Input: part model. Units: mm. Frame: model coordinates. Face numbers are marked on the shaded views. Round coordinates to 2 decimals unless told otherwise and drop trailing zeros. Loops run counter-clockwise (first coordinate to the right, second up) from the corner with the lowest first, then second, coordinate; pieces in that order, holes last. Notation, with made-up numbers: M 78,52 L 85,52 A36 cw 85,88 Z; hole C 77.5,13.5 d4. An arc over 180 degrees is marked long. Use one line per item in the form item = value. Start each with the question number.
Q1. First-contact query: P1, Ø2, axis at x = -1, y = -0.5, coming from the +Z side; P2, Ø1, axis at x = -2, y = 1.5, coming from the -Z side. Flat tips, straight axial feed; report the tip coordinate or a pass-through.
Q2. Section query A-A, the plane z = 0. Output: boundary loops of the cut face in (x, y) (3 decimals).
Q3. Section query B-B, the plane x = 0. Output: boundary loops of the cut face in (y, z) (3 decimals).
Q4. Section query C-C, the plane y = -1.5. Output: boundary loops of the cut face in (x, z).
Q5. Section query D-D, the plane y = 0.25. Output: boundary loops of the cut face in (x, z), and give its area (3 significant figures).
Q6. Ray query, line 1 along Z through (x, y) = (4.5, 2.5); line 2 along X through (y, z) = (-1.25, 2.5); line 3 along Z through (x, y) = (3.75, -1.5). Return the intervals inside material, ascending.
Q7. Mould query, pull axis Z, two halves, no side actions, for the marked faces 1 and 2. Classes: pulls with the +Z half, pulls with the -Z half, needs draft (parallel to the pull), parting line crosses it, or undercut.
```python
from build123d import *

# Parameters (mm, degrees)
SZKIC1_R                    = 8
DODANIE_WYCI_GNI_CIE1_DEPTH = 3.375
ZAOKR_GLENIE1_R             = 0.2


with BuildPart() as part:
    # Szkic1 → Dodanie-wyciągnięcie1 (new body, symmetric)
    with BuildSketch(Plane(origin=(0, 0, 0), x_dir=(1, 0, 0), z_dir=(0, 1, 0))):
        Circle(SZKIC1_R)
    extrude(amount=DODANIE_WYCI_GNI_CIE1_DEPTH, both=True)

    # Szkic3 → Wycięcie-obrót1 (revolve, cut)
    with BuildSketch(Plane.XY):
        with BuildLine():
            Line((0, -6.33), (0, 6.33))
            ThreePointArc((0, 6.33), (6.33, 0), (0, -6.33))
        make_face()
    revolve(axis=Axis((0, -6.33, 0), (0, 1, 0)), mode=Mode.SUBTRACT)

    # Zaokrąglenie1
    zaokr_glenie1_edges = [part.edges().sort_by_distance(p)[0] for p in [
        (-8, -3.375, 0),
        (-8, 3.375, 0),
    ]]
    fillet(zaokr_glenie1_edges, radius=ZAOKR_GLENIE1_R)


solid = part.part
```
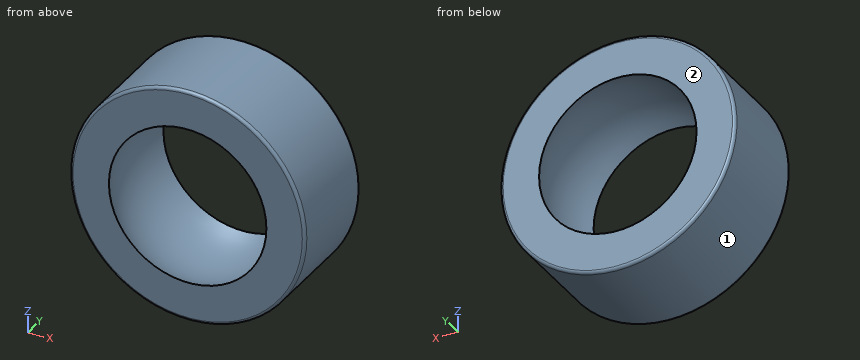
Results found:
q1.P1 = 8
q1.P2 = -7.86
q2.outline = M -8,-3.175 A0.2 ccw -7.8,-3.375 L -5.355,-3.375 A6.33 cw -5.355,3.375 L -7.8,3.375 A0.2 ccw -8,3.175 Z; M 5.355,-3.375 L 7.8,-3.375 A0.2 ccw 8,-3.175 L 8,3.175 A0.2 ccw 7.8,3.375 L 5.355,3.375 A6.33 cw Z
q3.outline = M -3.375,-7.8 A0.2 ccw -3.175,-8 L 3.175,-8 A0.2 ccw 3.375,-7.8 L 3.375,-5.355 A6.33 cw -3.375,-5.355 Z; M -3.375,5.355 A6.33 cw 3.375,5.355 L 3.375,7.8 A0.2 ccw 3.175,8 L -3.175,8 A0.2 ccw -3.375,7.8 Z
q4.outline = C 0,0 d16; hole C 0,0 d12.3
q5.outline = C 0,0 d16; hole C 0,0 d12.65
q5.area = 75.4 mm²
q6.line_1 = -6.61 to -3.68, 3.68 to 6.61
q6.line_2 = -7.6 to -5.68, 5.68 to 7.6
q6.line_3 = -7.07 to -4.87, 4.87 to 7.07
q7.face_1 = parting line crosses it
q7.face_2 = needs draft
